Source: CAD feature listing. Evaluate the final solid. Frame: model axes, mm. A direction names the side the tool comes from. Round coordinates to 2 decimals unless told otherwise and drop trailing zeros. Write each loop counter-clockwise with the first axis right and the second up, starting at its lowest first coordinate (ties: lowest second). Pieces come first, ordered by that corner, then holes.
from build123d import *

# Parameters (mm, degrees)
BOSS_EXTRUDE1_DEPTH = 1
SKETCH2_W           = 7.706049631
SKETCH2_H           = 13.7
BOSS_EXTRUDE2_DEPTH = 0.1
SKETCH3_R           = 0.478791287
CUT_EXTRUDE1_DEPTH  = 2.1
SKETCH4_W           = 5
SKETCH4_H           = 5
BOSS_EXTRUDE3_DEPTH = 1
SKETCH6_W           = 5.021657736
SKETCH6_H           = 2.270064456
BOSS_EXTRUDE5_DEPTH = 1


with BuildPart() as part:
    # Sketch1 → Boss-Extrude1 (new body)
    with BuildSketch(Plane.XY):
        with BuildLine():
            Line((13.817814776, 5.306721311), (13.817814776, 4.706721311))
            ThreePointArc((13.817814776, 4.706721311), (13.117814776, 4.006721311), (13.817814776, 3.306721311))
            Line((13.817814776, 3.306721311), (13.817814776, 2.706721311))
            ThreePointArc((13.817814776, 2.706721311), (13.117814776, 2.006721311), (13.817814776, 1.306721311))
            Line((13.817814776, 1.306721311), (13.817814776, 0.706721311))
            ThreePointArc((13.817814776, 0.706721311), (13.117814776, 0.006721311), (13.817814776, -0.693278689))
            Line((13.817814776, -0.693278689), (13.817814776, -1.293278689))
            ThreePointArc((13.817814776, -1.293278689), (13.117814776, -1.993278689), (13.817814776, -2.693278689))
            Line((13.817814776, -2.693278689), (13.817814776, -3.293278689))
            ThreePointArc((13.817814776, -3.293278689), (13.117814776, -3.993278689), (13.817814776, -4.693278689))
            Line((13.817814776, -4.693278689), (13.817814776, -5.793278689))
            Line((13.817814776, -5.793278689), (-9.482185224, -5.793278689))
            Line((-9.482185224, -5.793278689), (-9.482185224, 7.906721311))
            Line((-9.482185224, 7.906721311), (13.817814776, 7.906721311))
            Line((13.817814776, 7.906721311), (13.817814776, 6.706721311))
            ThreePointArc((13.817814776, 6.706721311), (13.117814776, 6.006721311), (13.817814776, 5.306721311))
        make_face()
    extrude(amount=BOSS_EXTRUDE1_DEPTH)

    # Sketch2 → Boss-Extrude2 (add)
    with BuildSketch(Plane.XY.offset(1)):
        with Locations((-5.629160408, 1.056721311)):
            Rectangle(SKETCH2_W, SKETCH2_H)
    extrude(amount=BOSS_EXTRUDE2_DEPTH)

    # Sketch3 → Cut-Extrude1 (cut)
    with BuildSketch(Plane.XY.offset(1.1)):
        with Locations((-5.982185224, 5.806721311)):
            Circle(SKETCH3_R)
    extrude(amount=-CUT_EXTRUDE1_DEPTH, mode=Mode.SUBTRACT)

    # Sketch4 → Boss-Extrude3 (add)
    with BuildSketch(Plane.XY.offset(1)):
        with Locations((6.317814776, 0.406721311)):
            Rectangle(SKETCH4_W, SKETCH4_H)
    extrude(amount=BOSS_EXTRUDE3_DEPTH)

    # Sketch6 → Boss-Extrude5 (add)
    with BuildSketch(Plane.XY.offset(1)):
        with Locations((3.555076388, 5.367550784)):
            Rectangle(SKETCH6_W, SKETCH6_H)
    extrude(amount=BOSS_EXTRUDE5_DEPTH)


solid = part.part
1) Section query A-A on z = 1.4. Return the cut outline in (x, y), then the cut area to 3 significant figures.
Taken from the geometry:
outline: (1.04, 4.23) - (6.07, 4.23) - (6.07, 6.5) - (1.04, 6.5) - close; (3.82, -2.09) - (8.82, -2.09) - (8.82, 2.91) - (3.82, 2.91) - close
area: 36.4 mm2
2) Section query D-D on z = 0.45. Return the cut outline in (x, y).
Taken from the geometry:
outline: (-9.48, -5.79) - (13.82, -5.79) - (13.82, -4.69) arc R0.7 cw to (13.82, -3.29) - (13.82, -2.69) arc R0.7 cw to (13.82, -1.29) - (13.82, -0.69) arc R0.7 cw to (13.82, 0.71) - (13.82, 1.31) arc R0.7 cw to (13.82, 2.71) - (13.82, 3.31) arc R0.7 cw to (13.82, 4.71) - (13.82, 5.31) arc R0.7 cw to (13.82, 6.71) - (13.82, 7.91) - (-9.48, 7.91) - close; hole circle Ø0.96 at (-5.98, 5.81)
3) Contact query for flat-ended pins moving along their axis: P1, Ø2.5, axis at x = -5.5, y = -2, coming from the +Z side; P2, Ø0.5, axis at x = 6.5, z = 1.5, coming from the -Y side; P3, Ø0.8, axis at x = 5.5, z = 1.5, coming from the +Y side. Output: stop coordinate, or through.
Taken from the geometry:
P1: stops at z = 1.1
P2: stops at y = -2.09
P3: stops at y = 6.5
4) Material intervals for line 1 (X direction, y = 4.75, z = 1.75); line 2 (Z direction, x = 10.25, y = -1.25); line 3 (Z direction, x = -5.75, y = 1.5), sorted ascending.
Taken from the geometry:
line 1: x = 1.04 to 6.07
line 2: z = 0 to 1
line 3: z = 0 to 1.1
5) Section query C-C on y = 1.75. Return the cut outline in (x, z).
Taken from the geometry:
outline: (-9.48, 0) - (13.17, 0) - (13.17, 1) - (8.82, 1) - (8.82, 2) - (3.82, 2) - (3.82, 1) - (-1.78, 1) - (-1.78, 1.1) - (-9.48, 1.1) - close
6) Section query B-B on x = 7. Return the cut outline in (y, z).
Taken from the geometry:
outline: (-5.79, 0) - (7.91, 0) - (7.91, 1) - (2.91, 1) - (2.91, 2) - (-2.09, 2) - (-2.09, 1) - (-5.79, 1) - close
7) Pull-direction query (X, two-part tool) for faces 5 (the face through (13.118, 0.022, 0.493)), 6 (the face through (6, 4, 1)), 7 (the face through (2, -5.793, 0.5)), 8 (the face through (-9.482, 1, 0.5)); classes: released by +X, released by -X, zero draft, split by the parting line, or undercut.
Taken from the geometry:
face 5: released by +X
face 6: undercut
face 7: zero draft
face 8: released by -X
8) Reachability of faces 1 (the face through (13.818, 7.3, 0.5)), 2 (the face through (6.066, 5.4, 1.5)), 3 (the face through (8.818, 0.4, 1.5)), 4 (the face through (-6, 1, 1.1)) from +Z, -Z, +X, -X, +Y, -Y: full face, straight path, thin tool, end or side. Return the list, or none.
Taken from the geometry:
face 1: +Z, -Z, +X, +Y, -Y
face 2: +Z, +X, +Y
face 3: +Z, +X, +Y, -Y
face 4: +Z, -X, +Y, -Y
